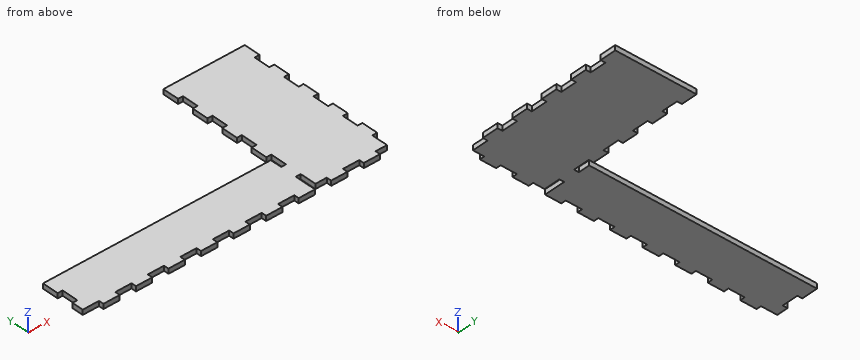
from build123d import *

# Parameters (mm, degrees)
BOSS_EXTRUDE1_DEPTH = 6
SKETCH2_W           = 20
SKETCH2_H           = 6
CUT_EXTRUDE1_DEPTH  = 10
LPATTERN1_COUNT     = 10
LPATTERN1_PITCH     = 40
SKETCH3_W           = 6
SKETCH3_H           = 20
CUT_EXTRUDE2_DEPTH  = 10
SKETCH4_W           = 6
SKETCH4_H           = 20
CUT_EXTRUDE3_DEPTH  = 10
LPATTERN2_COUNT     = 5
LPATTERN2_PITCH     = 40
SKETCH5_W           = 6
SKETCH5_H           = 20
CUT_EXTRUDE4_DEPTH  = 10
LPATTERN3_COUNT     = 5
LPATTERN3_PITCH     = 40


with BuildPart() as part:
    # Sketch1 → Boss-Extrude1 (new body)
    with BuildSketch(Plane.XY):
        Polygon((-220.231213873, -93.901734104), (59.768786127, -93.901734104), (59.768786127, 52.098265896), (159.768786127, 52.098265896), (159.768786127, -153.901734104), (59.768786127, -153.901734104), (-220.231213873, -153.901734104), align=None)
    extrude(amount=BOSS_EXTRUDE1_DEPTH)

    # Sketch2 → Cut-Extrude1 (cut)
    with BuildSketch(Plane.XY.offset(6)):
        with Locations((-210.231213873, -150.901734104)):
            Rectangle(SKETCH2_W, SKETCH2_H)
    cut_extrude1 = extrude(amount=-CUT_EXTRUDE1_DEPTH, mode=Mode.SUBTRACT)

    # LPattern1: Cut-Extrude1 ×10
    with Locations(*[(i * LPATTERN1_PITCH, 0, 0) for i in range(1, LPATTERN1_COUNT)]):
        add(cut_extrude1, mode=Mode.SUBTRACT)

    # Sketch3 → Cut-Extrude2 (cut)
    with BuildSketch(Plane.XY.offset(6)):
        with Locations((-217.231213873, -123.901734104)):
            Rectangle(SKETCH3_W, SKETCH3_H)
    extrude(amount=-CUT_EXTRUDE2_DEPTH, mode=Mode.SUBTRACT)

    # Sketch4 → Cut-Extrude3 (cut)
    with BuildSketch(Plane.XY.offset(6)):
        with Locations((156.768786127, 22.098265896)):
            Rectangle(SKETCH4_W, SKETCH4_H)
    cut_extrude3 = extrude(amount=-CUT_EXTRUDE3_DEPTH, mode=Mode.SUBTRACT)

    # LPattern2: Cut-Extrude3 ×5
    with Locations(*[(0, -i * LPATTERN2_PITCH, 0) for i in range(1, LPATTERN2_COUNT)]):
        add(cut_extrude3, mode=Mode.SUBTRACT)

    # Sketch5 → Cut-Extrude4 (cut)
    with BuildSketch(Plane.XY.offset(6)):
        with Locations((62.768786127, 22.098265896)):
            Rectangle(SKETCH5_W, SKETCH5_H)
    cut_extrude4 = extrude(amount=-CUT_EXTRUDE4_DEPTH, mode=Mode.SUBTRACT)

    # LPattern3: Cut-Extrude4 ×5
    with Locations(*[(0, -i * LPATTERN3_PITCH, 0) for i in range(1, LPATTERN3_COUNT)]):
        add(cut_extrude4, mode=Mode.SUBTRACT)


solid = part.part
Can you work these out from the model? Positions are in its coordinate system, mm. Coordinates: 2 decimals unless noted, no trailing zeros. Write each loop counter-clockwise with the first axis right and the second up, starting at its lowest first coordinate (ties: lowest second). Pieces come first, ordered by that corner, then holes. Notation, with made-up numbers: (84.5, 13) -> (106.5, 13) arc R4 cw to (106.5, 19) -> close; hole circle Ø10 at (8, -37.75). An arc over 180 degrees is marked (long way). Write each question's results on one line, items separated by ' | '. Start each with the question number.
Item 1: If we section it at A-A, the plane x = -149.5: Write out the boundary of the cut face in (y, z), and give its area (3 significant figures).
Item 2: Please list where these lines run through material, in increasing order: probe 1 along X at (y, z) = (-128.5, 5.6); probe 2 along X at (y, z) = (-52.5, 0.3); probe 3 along Y at (x, z) = (-65.5, 4.75).
Item 3: I'm going to push flat-ended pins straight in: P1, Ø1, axis at x = -123, z = 5, coming from the -Y side; P2, Ø1.8, axis at x = 62.5, z = 4, coming from the -Y side; P3, Ø3, axis at y = -150, z = 1.5, coming from the +X side. Where does each tip first touch, or does it pass through?
Item 4: If we section it at B-B, the plane y = -76: Write out the boundary of the cut face in (x, z), and give its area (3 significant figures).
Answer block:
1) outline: (-153.9, 0) -> (-93.9, 0) -> (-93.9, 6) -> (-153.9, 6) -> close | area: 360 mm²
2) probe 1: -214.23 to 59.77, 65.77 to 153.77 | probe 2: 65.77 to 153.77 | probe 3: -153.9 to -93.9
3) P1: y = -147.9 | P2: y = -127.9 | P3: x = 139.77
4) outline: (59.77, 0) -> (159.77, 0) -> (159.77, 6) -> (59.77, 6) -> close | area: 600 mm²
